from build123d import *

# Parameters (mm, degrees)
F1_DEPTH     = 5
F3_DEPTH     = 25
F4_T1_DEPTH  = 5.9478639207
F4_T6_DEPTH  = 11.0004984696
F4_T11_DEPTH = 3.281815708
F4_T16_DEPTH = 7.2643009793
F4_T21_DEPTH = 5.7529029378
F5_T1_DEPTH  = 7.6329796459
F5_T3_DEPTH  = 7.4610000963
F5_T8_DEPTH  = 7.4842482227
F5_T13_DEPTH = 7.4842482227
F5_T18_DEPTH = 3.281815708
F5_T23_DEPTH = 11.0004984696


# Not quite as in the source:
# - a fillet or chamfer that OpenCascade refuses, or shapes differently, is made with other operations: its cross-section is extruded or revolved along the edge and cut away or added


with BuildPart() as f1:
    # F0 (on Front) → F1 (new body)
    with BuildSketch(Plane.XZ):
        Polygon((-7.11, 0), (0, 0), (0, 0.85), (-7.3617814707, 0.85), (-12.2206721932, -2.3054005297), (-20.7425294551, -21.4458053218), (-19.9660158161, -21.7915314684), (-11.5465673044, -2.8811404952), align=None)
    extrude(amount=F1_DEPTH)

    # F2 (on face) → F3 (cut)
    with BuildSketch(Plane(origin=(-8.5658121179, 0, 3.8137452678), x_dir=(0, 1, 0), z_dir=(0.9135454576, 0, -0.4067366431))):
        Polygon((-4, -14.4284648367), (-5, -7.3284648367), (-5, -28.0284648367), (-2, -28.0284648367), (-3, -17.2284648367), align=None)
    extrude(amount=-F3_DEPTH, mode=Mode.SUBTRACT)

    # F4: chamfer of 0.03 on 5 edges, made by hand

    # F4_s2 → F4_t1 (cut)
    with BuildSketch(Plane(origin=(-4.7250832121, 0, -3.0685049164), x_dir=(0, 1, 0), z_dir=(-0.8386705679, 0, -0.544639035))):
        Polygon((-4.97, -4.722383539), (-5, -4.692383539), (-5, -4.722383539), align=None)
    extrude(amount=F4_T1_DEPTH, mode=Mode.SUBTRACT)


with BuildPart() as f4_tool4:
    # F4_s5 → F4_t6 (new body)
    with BuildSketch(Plane(origin=(-11.2598610976, 2.5632795791, -25.2900620943), x_dir=(0.2219685938, 0.9750538156, 0), z_dir=(0.4050042191, -0.0921982106, 0.9096543698))):
        Polygon((-6.352559346, 8.2598889374), (-6.3880194376, 8.283182325), (-6.3819360855, 8.2538055854), align=None)
    extrude(amount=F4_T6_DEPTH)

    split(bisect_by=Plane(origin=(-0.3055183915, 0.3704168412, 0.2808368777), x_dir=(0.771450463, 0.6362893863, 0), z_dir=(0.549241742, -0.6659120918, -0.5048708694)), keep=Keep.TOP)


with BuildPart() as f1_1:
    add(f1.part)

    # F4_t3: cut F4_tool4
    add(f4_tool4.part, mode=Mode.SUBTRACT)


with BuildPart() as f4_tool9:
    # F4_s10 → F4_t11 (new body)
    with BuildSketch(Plane(origin=(-5.8578101844, 5.1435618144, -13.1568570886), x_dir=(0.659809773, 0.751432674, 0), z_dir=(0.3830409438, -0.336336397, 0.8603240456))):
        Polygon((-12.5057496784, 2.3040031535), (-12.5477702003, 2.3098577021), (-12.5296872137, 2.2859201669), align=None)
    extrude(amount=F4_T11_DEPTH)

    split(bisect_by=Plane(origin=(-2.1159962098, 2.405108563, 1.1858724964), x_dir=(0.7507908153, 0.6605400454, 0), z_dir=(0.6194574075, -0.7040949829, -0.3471639027)), keep=Keep.TOP)


with BuildPart() as f1_2:
    add(f1_1.part)

    # F4_t8: cut F4_tool9
    add(f4_tool9.part, mode=Mode.SUBTRACT)


with BuildPart() as f4_tool14:
    # F4_s15 → F4_t16 (new body)
    with BuildSketch(Plane.YZ.offset(-7.1871504896)):
        Polygon((-4.97, 0), (-5, 0.03), (-5, 0), align=None)
    extrude(amount=F4_T16_DEPTH)

    split(bisect_by=Plane(origin=(0.2989023851, -0.5488082305, -0.4602693104), x_dir=(0.878196468, 0.4783000769, 0), z_dir=(0.385117955, -0.7071067812, -0.5930296458)), keep=Keep.TOP)


with BuildPart() as f1_3:
    add(f1_2.part)

    # F4_t13: cut F4_tool14
    add(f4_tool14.part, mode=Mode.SUBTRACT)


with BuildPart() as f4_tool19:
    # F4_s20 → F4_t21 (new body)
    with BuildSketch(Plane(origin=(-9.7610352954, 0, -6.3388904383), x_dir=(0, 1, 0), z_dir=(0.8386705679, 0, 0.544639035))):
        Polygon((-4.97, 3.872383539), (-5, 3.902383539), (-5, 3.872383539), align=None)
    extrude(amount=F4_T21_DEPTH)

    split(bisect_by=Plane(origin=(-8.5658121179, 0, 3.8137452678), x_dir=(0, 1, 0), z_dir=(0.9135454576, 0, -0.4067366431)), keep=Keep.TOP)

    split(bisect_by=Plane(origin=(0, -2.485, -2.485), x_dir=(1, 0, 0), z_dir=(0, -0.7071067812, -0.7071067812)), keep=Keep.TOP)


with BuildPart() as f1_4:
    add(f1_3.part)

    # F4_t18: cut F4_tool19
    add(f4_tool19.part, mode=Mode.SUBTRACT)

    # F5: chamfer of 0.03 on 5 edges, made by hand

    # F5_s2 → F5_t1 (cut)
    with BuildSketch(Plane(origin=(-5.6229623165, 1.9471236166, -12.6293801411), x_dir=(0.3272176494, 0.9449489986, 0), z_dir=(0.4027614046, -0.1394685218, 0.9046169258))):
        Polygon((-8.7284463039, 7.9822536907), (-8.7481067262, 7.9446575766), (-8.7570745721, 7.9732858448), align=None)
    extrude(amount=F5_T1_DEPTH, mode=Mode.SUBTRACT)

    # F5_s4 → F5_t3 (cut)
    with BuildSketch(Plane.YZ.offset(-7.3838496067)):
        Polygon((-4.97, 0.85), (-5, 0.82), (-5, 0.85), align=None)
    extrude(amount=F5_T3_DEPTH, mode=Mode.SUBTRACT)


with BuildPart() as f5_tool6:
    # F5_s7 → F5_t8 (new body)
    with BuildSketch(Plane(origin=(-5.5630590396, 1.9263802648, -12.4948351783), x_dir=(0.3272176494, 0.9449489986, 0), z_dir=(0.4027614046, -0.1394685218, 0.9046169258))):
        Polygon((-8.4743573363, 7.1711194253), (-8.5119534504, 7.1907798476), (-8.5029856044, 7.1621515794), align=None)
    extrude(amount=F5_T8_DEPTH)

    split(bisect_by=Plane(origin=(0.2989023851, -0.5488082305, -0.4602693104), x_dir=(0.878196468, 0.4783000769, 0), z_dir=(0.385117955, -0.7071067812, -0.5930296458)), keep=Keep.TOP)


with BuildPart() as f1_5:
    add(f1_4.part)

    # F5_t5: cut F5_tool6
    add(f5_tool6.part, mode=Mode.SUBTRACT)


with BuildPart() as f5_tool11:
    # F5_s12 → F5_t13 (new body)
    with BuildSketch(Plane(origin=(-5.5630590396, 1.9263802648, -12.4948351783), x_dir=(0.3272176494, 0.9449489986, 0), z_dir=(0.4027614046, -0.1394685218, 0.9046169258))):
        Polygon((-8.4743573363, 7.1711194253), (-8.5119534504, 7.1907798476), (-8.5029856044, 7.1621515794), align=None)
    extrude(amount=F5_T13_DEPTH)

    split(bisect_by=Plane(origin=(-2.1090512339, 0, 3.2476541019), x_dir=(0, 1, 0), z_dir=(0.544639035, 0, -0.8386705679)), keep=Keep.TOP)


with BuildPart() as f1_6:
    add(f1_5.part)

    # F5_t10: cut F5_tool11
    add(f5_tool11.part, mode=Mode.SUBTRACT)


with BuildPart() as f5_tool16:
    # F5_s17 → F5_t18 (new body)
    with BuildSketch(Plane(origin=(-5.8578101844, 5.1435618144, -13.1568570886), x_dir=(0.659809773, 0.751432674, 0), z_dir=(0.3830409438, -0.336336397, 0.8603240456))):
        Polygon((-13.0181009663, 2.9822333193), (-13.0239555149, 2.9402127974), (-13.0420385015, 2.9641503327), align=None)
    extrude(amount=F5_T18_DEPTH)

    split(bisect_by=Plane(origin=(-7.0244742563, -7.3545925713, 2.3820711564), x_dir=(0.7231501661, -0.6906908406, 0), z_dir=(-0.6724909686, -0.7040949829, 0.2280485743)), keep=Keep.TOP)


with BuildPart() as f1_7:
    add(f1_6.part)

    # F5_t15: cut F5_tool16
    add(f5_tool16.part, mode=Mode.SUBTRACT)


with BuildPart() as f5_tool21:
    # F5_s22 → F5_t23 (new body)
    with BuildSketch(Plane(origin=(-11.2598610976, 2.5632795791, -25.2900620943), x_dir=(0.2219685938, 0.9750538156, 0), z_dir=(0.4050042191, -0.0921982106, 0.9096543698))):
        Polygon((-6.5249209865, 9.0922298921), (-6.548214374, 9.0567698005), (-6.554297726, 9.0861465401), align=None)
    extrude(amount=F5_T23_DEPTH)

    split(bisect_by=Plane(origin=(-9.881776244, -8.860018193, 0.9359011948), x_dir=(0.6675656779, -0.7445509155, 0), z_dir=(-0.742706634, -0.6659120918, 0.0703416075)), keep=Keep.TOP)


with BuildPart() as f1_8:
    add(f1_7.part)

    # F5_t20: cut F5_tool21
    add(f5_tool21.part, mode=Mode.SUBTRACT)


solid = f1_8.part
For this review, take the finished solid that the model builds, in its own axes (mm). A direction names the side the tool comes from. Round coordinates to 2 decimals unless told otherwise and drop trailing zeros. Order: outer loops, then holes, each group sorted by start corner. A loop starts at its lowest first (then second) coordinate and runs counter-clockwise, first axis right, second up. Notation, with made-up numbers: M -35,61 L 20,61 A27 ccw 20,90 Z; hole C -2.75,-23.75 d4. An arc over 180 degrees is marked long. Write each question's results on one line, items separated by ' | '. Start each with the question number.
1. Add section C-C (z = -6.75). State the section outline as (x, y) points, then the cut area to 3 significant figures.
2. Add section A-A (x = -1.5). State the section outline as (y, z) points.
3. Clearance check with flat-ended pins moving along their axes: pin 1 Ø1 at (y, z) = (-2, -5.5) entering from +X; pin 2 Ø1.5 at (y, z) = (-2, -15) entering from +X; pin 3 Ø6 at (x, z) = (-9, -11) entering from +Y. State where each tip first meets the part, or that it passes through.
4. Add section B-B (y = -3.55). State the section outline as (x, z) points, then the cut area to 3 significant figures.
5. To check wall thickness, follow L1, parallel to Z at x = -3.75, y = -4.05; L2, parallel to X at y = -2.2, z = -12.25; L3, parallel to Z at x = -9.75, y = -2.85. State the ranges of each line that lie inside material, in increasing order. Write a range as [from, to].
6. Tool access review of faces 1 (the face through (-4, -2, 0.85)), 2 (the face through (-4, -2, 0)): name each direction out of +Z, -Z, +X, -X, +Y, -Y from which nothing blocks a thin tool from reaching the whole face with its end or side.
Output values:
1) outline: M -14.2,-4.32 L -14.17,-4.35 L -13.3,-4.4 L -13.27,-4.37 L -13.27,0 L -14.2,0 Z | area: 4.07 mm^2
2) outline: M -5,0.03 L -4.97,0 L 0,0 L 0,0.85 L -4.97,0.85 L -5,0.82 Z
3) pin 1: x = -12.49 | pin 2: x = -16.61 | pin 3: through
4) outline: M -15.7,-10.18 L -14.97,-10.51 L -14.91,-10.44 L -11.55,-2.88 L -7.11,0 L 0,0 L 0,0.85 L -7.36,0.85 L -12.22,-2.31 L -15.69,-10.09 Z | area: 18.1 mm^2
5) L1: [0, 0.85] | L2: [-16.65, -15.72] | L3: [-1.71, -0.7]
6) face 1: +Z, +X, -X, +Y, -Y | face 2: -Z, +X, +Y, -Y
